Autodesk Inventor part; units mm, degrees
ref_plane "YZ Plane" through (0, 0, 0) normal (1, 0, 0) x (0, 1, 0)
ref_plane "XZ Plane" through (0, 0, 0) normal (0, 1, 0) x (-1, 0, 0)
ref_plane "XY Plane" through (0, 0, 0) normal (0, 0, 1) x (1, 0, 0)
sketch "Sketch1" plane through (0, 0, 0) normal (1, 0, 0) x (0, 1, 0)
  line L0 (0, 16) -> (2.5, 16) construction
  arc A0 (9.9609, 0) -> (2.5, 16) centre (-28.1983, -8.0544) ccw construction
  line L1 (0, 12) -> (0, 0) construction
  line L2 (2.5, 16) -> (2.5, 16) construction
  line L3 (9.9609, 0) -> (4.5, 0) construction
  line L4 (4.5, 9) -> (0, 9)
  line L5 (4.5, 9) -> (4.5, 0)
  line L6 (0, 12) -> (0, 9)
  line L7 (9.9609, 0) -> (2.5, 16) construction
  line L8 (3.2, 14.4988) -> (3.2, 16)
  line L9 (3.2, 16) -> (2.5, 16)
  line L10 (7, 0) -> (7, 6.3497)
  line L11 (4.5, 0) -> (7, 0)
  line L12 (7, 6.3497) -> (3.2, 14.4988)
  line L13 (0, 12) -> (0.8, 12)
  line L14 (0.8, 12) -> (0.8, 16)
  line L15 (2.5, 16) -> (0.8, 16)
  dimension "d0" = 2.5
  dimension "d5" = 4.5
  dimension "d11" = 9
  dimension "d12" = 16
  dimension "d13" = 115
  dimension "d14" = 3.2
  dimension "d18" = 1.5011
  dimension "d19" = 8.1491
  dimension "d20" = 7
  dimension "d21" = 4
  dimension "d22" = 0.8
revolve "Revolution1" add sketch "Sketch1" angle 360 about axis through (0, 0, 12) along (0, 0, -1)
sketch "Sketch2" plane through (0, 0, 0) normal (1, 0, 0) x (0, 1, 0)
  arc A0 (-2.5, 15) -> (2.5, 15) centre (0, 15) ccw
  circle A1 centre (0, 15) radius 1.5
  line L0 (0.6744, 16.3398) -> (-0.6744, 13.6602)
  point P0 (0, 0)
  dimension "d8" = 3
revolve "Revolution2" [suppressed]
fillet "Fillet1" radius 0.5 2 edges at (0, -3.2, 16) (0, -4.5, 9)
properties part number "brush fitting parta"
Work out the finished part from the listing and answer in its coordinate system (mm). A direction names the side the tool comes from. Coordinates: 2 decimals unless noted, no trailing zeros. Write each loop counter-clockwise with the first axis right and the second up, starting at its lowest first coordinate (ties: lowest second). Pieces come first, ordered by that corner, then holes. Notation, with made-up numbers: M -4.5,67 L 27.5,67 A19 cw 27.5,97 Z; hole C 77.25,-18 d11. An arc over 180 degrees is marked long. Answer as CSV lines item,"result". Start each with the question number.
Item 1: Determine the mould class of faces 4 (the face through (-1, -1, 16)), 5 (the face through (1.947, -2.539, 15.006)), 6 (the face through (0.49, -0.63, 14.03)), 7 (the face through (4.46, -0.59, 4.19)) for opening direction X: released by +X, released by -X, zero draft, split by the parting line, or undercut.
Item 2: A tool of negligible diameter and unlimited length cuts with its end or side. For faces 1 (the face through (-5, 0, 0)), 2 (the face through (0, 0, 12)), 3 (the face through (0, 0, 9)), from which of +Z, -Z, +X, -X, +Y, -Y can it reach the whole face along a straight path? Write none if from no direction.
Item 3: Section A-A on x = 0 is taken. Write down the section's boundary in (y, z), and give its area (3 significant figures).
Item 4: Section D-D on z = 10.5 is taken. Write down the section's boundary in (x, y), and give its area (3 significant figures).
Item 5: Flat-ended cylindrical pins translate along their axes: P1, Ø3, axis at y = 0.5, z = 12, coming from the -X side; P2, Ø4, axis at y = 3, z = 11, coming from the +X side; P3, Ø1.3, axis at x = 0, y = 0, coming from the +Z side. Find the tip coordinate at first contact, or state that the pin passes through.
Item 6: Consider L1, parallel to X at y = 0, z = 3.5; L2, parallel to Y at x = -0.5, z = 3; L3, parallel to X at y = 2, z = 2.75. Determine where each line is inside the solid, lowest interval first.
Item 7: Section C-C on z = 3 is taken. Write down the section's boundary in (x, y).
Checks:
1,face 4,"zero draft"
1,face 5,"split by the parting line"
1,face 6,"undercut"
1,face 7,"undercut"
2,face 1,"-Z, +X, -X, +Y, -Y"
2,face 2,"+Z"
2,face 3,"-Z"
3,outline,"M -7,0 L -4.5,0 L -4.5,8.5 A0.5 cw -4,9 L 4,9 A0.5 cw 4.5,8.5 L 4.5,0 L 7,0 L 7,6.35 L 3.2,14.5 L 3.2,15.5 A0.5 ccw 2.7,16 L 0.8,16 L 0.8,12 L -0.8,12 L -0.8,16 L -2.7,16 A0.5 ccw -3.2,15.5 L -3.2,14.5 L -7,6.35 Z"
3,area,"94.2 mm²"
4,outline,"C 0,0 d10.13"
4,area,"80.6 mm²"
5,P1,"stops at x = -5.05"
5,P2,"stops at x = 5.28"
5,P3,"stops at z = 12"
6,L1,"x = -7 to -4.5, 4.5 to 7"
6,L2,"y = -6.98 to -4.47, 4.47 to 6.98"
6,L3,"x = -6.71 to -4.03, 4.03 to 6.71"
7,outline,"C 0,0 d14; hole C 0,0 d9"
